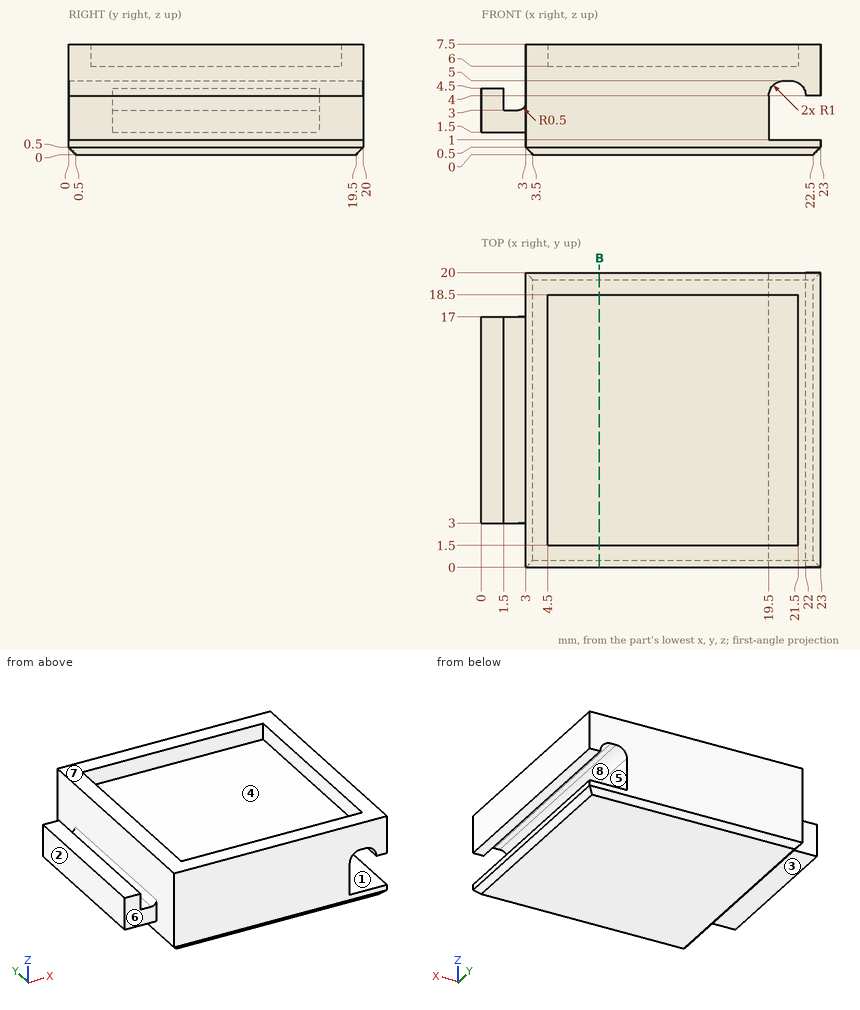
Source: three-view drawing plus pictorial views. Frame: mm from the lowest corner of the part. A direction names the side the tool comes from. Round coordinates to 2 decimals unless told otherwise and drop trailing zeros. Loops run counter-clockwise (first coordinate to the right, second up) from the corner with the lowest first, then second, coordinate; pieces in that order, holes last.
Q1. Section B-B, the plane x = 8. Return loops of the section in (y, z), plus the area to 3 significant figures.
Q2. First-contact query: P1, Ø2.5, axis at x = 1.5, z = 3, coming from the +Y side; P2, Ø0.8, axis at x = 2, y = 10.5, coming from the +Z side; P3, Ø1.6, axis at x = 0.5, y = 10, coming from the +Z side. Flat tips, straight axial feed; report the tip coordinate or a pass-through.
Q3. Mould query, pull axis Z, two halves, no side actions, for the marked faces 1, 2, 3 and 4. Classes: pulls with the +Z half, pulls with the -Z half, needs draft (parallel to the pull), parting line crosses it, or undercut.
Q4. Ray query, line 1 (X direction, y = 3, z = 7); line 2 (Y direction, x = 11.5, z = 6.75); line 3 (X direction, y = 16.75, z = 3.75). Return the intervals inside material, ascending.
Q5. Access query for the marked faces 5, 6, 7 and 8. Directions: +Z, -Z, +X, -X, +Y, -Y. A direction counts if a zero-diameter tool reaches every point of the face in a straight line with its end or side. Return the directions, or none.
Solutions:
1. outline: (0, 0.5) - (0.5, 0) - (19.5, 0) - (20, 0.5) - (20, 7.5) - (18.5, 7.5) - (18.5, 6) - (1.5, 6) - (1.5, 7.5) - (0, 7.5) - close
1. area: 124 mm2
2. P1: stops at y = 17
2. P2: stops at z = 3
2. P3: stops at z = 4.5
3. face 1: undercut
3. face 2: needs draft
3. face 3: pulls with the -Z half
3. face 4: pulls with the +Z half
4. line 1: x = 3 to 4.5, 21.5 to 23
4. line 2: y = 0 to 1.5, 18.5 to 20
4. line 3: x = 0 to 1.5, 3 to 19.5
5. face 5: +X, +Y, -Y
5. face 6: +Z, -Z, -X, -Y
5. face 7: +Z, +X, -X, +Y, -Y
5. face 8: +Y, -Y
